Could you check a few things on this model? Use its own coordinates, in mm. Face numbers are marked on the shaded views. Coordinates: 2 decimals unless noted, no trailing zeros. Order: outer loops, then holes, each group sorted by start corner. A loop starts at its lowest first (then second) coordinate and runs counter-clockwise, first axis right, second up. Notation, with made-up numbers: (40.5, 1.5) -> (78.5, 1.5) arc R24 cw to (78.5, 24.5) -> close; hole circle Ø8 at (-25, 45). An arc over 180 degrees is marked (long way). Put each result on its own line as item: value. Start each with the question number.
Q1. If we section it at A-A (y = 0): Please give me the cut outline in (x, z) (3 decimals).
Q2. Will this pin go through, and if not, where does the flat tip stop? pin 1 (1 mm diameter, centred on y = 1, z = 21.5, fed in from -X).
Q3. We'd pull the mould along X, two halves only. Please class the marked faces 1, 2 and 3: +X half, -X half, draft (parallel to the pull), parting line (faces both ways), or undercut.
Q4. Please list where these lines run through material, in increasing order: line 1 along Y through (x, z) = (0, 22.1) (3 decimals); line 2 along Y through (x, z) = (-0.75, 22.5).
Q5. If we section it at C-C (z = 22): Please give me the cut outline in (x, y) (3 decimals), and give its area (3 significant figures).
Q6. If we section it at D-D (x = 2.5): Please give me the cut outline in (y, z), and give its area (3 significant figures).
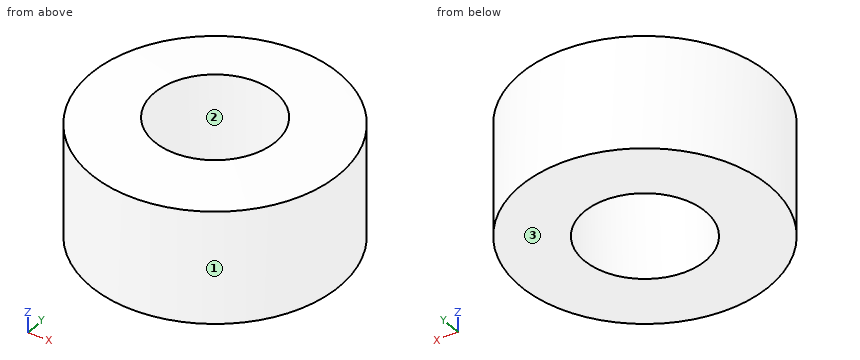
Autodesk Inventor part; units mm, degrees
ref_plane "Work Plane1" through (0, 0, 19.9) normal (0, 0, 1) x (1, 0, 0)
ref_plane "YZ Plane" through (0, 0, 0) normal (1, 0, 0) x (0, 1, 0)
ref_plane "XZ Plane" through (0, 0, 0) normal (0, 1, 0) x (-1, 0, 0)
sketch "Sketch1" plane through (0, 0, 0) normal (0, 0, 1) x (1, 0, 0)
  line L0 (-34.9979, 0) -> (51.0758, 0)
  arc A0 (23, 0) -> (-23, 0) centre (0, 0) ccw
  dimension "d0" = 46
revolve "Revolution1" add sketch "Sketch1" angle 360 about axis through (-34.9979, 0, 0) along (1, 0, 0)
ref_plane "Work Plane1" through (0, 0, 19.9) normal (0, 0, 1) x (1, 0, 0)
sketch "Sketch2" plane through (0, 0, 19.9) normal (0, 0, 1) x (1, 0, 0)
  circle A0 centre (0, 0) radius 11.5321
extrude "Extrusion1" cut sketch "Sketch2" against normal through all
sketch "Sketch3" plane through (0, 0, 19.9) normal (0, 0, 1) x (1, 0, 0)
  circle A0 centre (0, 0) radius 27.1797
extrude "Extrusion2" cut sketch "Sketch3" against normal through all
sketch "Sketch4" plane through (0, 0, 19.9) normal (0, 0, 1) x (1, 0, 0)
  circle A0 centre (0, 0) radius 1.55
  dimension "d9" = 3.1
extrude "Extrusion3" cut sketch "Sketch4" along normal through all
sketch "Sketch5" plane through (0, 0, 19.9) normal (0, 0, -1) x (-1, 0, 0)
  circle A0 centre (0, 0) radius 11.5321
  circle A1 centre (0, 0) radius 3.175
  dimension "d13" = 6.35
extrude "Extrusion4" cut sketch "Sketch5" against normal through all
properties part number "PVC Spacer"
The answers:
1. outline: (-3.175, 19.9) -> (-1.55, 19.9) -> (-1.55, 22.948) arc R23 ccw to (-3.175, 22.78) -> close; (1.55, 19.9) -> (3.175, 19.9) -> (3.175, 22.78) arc R23 ccw to (1.55, 22.948) -> close
2. pin 1: x = -3.14
3. face 1: parting line
3. face 2: undercut
3. face 3: draft
4. line 1: -3.175 to -1.55, 1.55 to 3.175
4. line 2: -3.09 to -1.36, 1.36 to 3.09
5. outline: circle Ø6.35 at (0, 0); hole circle Ø3.1 at (0, 0)
5. area: 24.1 mm^2
6. outline: (-1.96, 19.9) -> (1.96, 19.9) -> (1.96, 22.78) arc R22.86 ccw to (-1.96, 22.78) -> close
6. area: 11.5 mm^2
